Autodesk Inventor part; units mm, degrees
ref_plane "YZ Plane" through (0, 0, 0) normal (1, 0, 0) x (0, 1, 0)
ref_plane "XZ Plane" through (0, 0, 0) normal (0, 1, 0) x (-1, 0, 0)
ref_plane "XY Plane" through (0, 0, 0) normal (0, 0, 1) x (1, 0, 0)
sketch "Sketch1" plane through (0, 0, 0) normal (0, 0, 1) x (1, 0, 0)
  line L0 (107.2618, 7.9599) -> (127.2618, 7.9599)
  line L1 (127.2618, 7.9599) -> (127.2618, 2.9599)
  line L2 (127.2618, 2.9599) -> (107.2618, 2.9599)
  line L3 (107.2618, 2.9599) -> (107.2618, 7.9599)
  circle A0 centre (-95.9382, -3.1699) radius 7.5
  circle A1 centre (-95.9382, -3.1699) radius 10
  line L4 (-95.9382, -13.1699) -> (-67.2988, -13.1699)
  line L5 (-67.2988, -13.1699) -> (17.5278, -13.1699)
  line L6 (107.2618, 2.9599) -> (17.5278, -13.1699)
  line L7 (-95.9382, 6.8301) -> (17.5278, 6.8301)
  line L8 (17.5278, 6.8301) -> (107.2618, 7.9599)
  line L9 (-105.7312, -1.1457) -> (-107.876, -1.1457)
  line L10 (-109.876, -3.1457) -> (-109.876, -3.9908)
  line L11 (-107.876, -5.9908) -> (-105.5321, -5.9908)
  arc A2 (-107.876, -1.1457) -> (-109.876, -3.1457) centre (-107.876, -3.1457) ccw
  arc A3 (-109.876, -3.9908) -> (-107.876, -5.9908) centre (-107.876, -3.9908) ccw
  point P0 (0, 0)
  point P1 (107.2618, 5.4599)
  point P2 (-109.876, -5.9908)
  point P3 (-109.876, -1.1457)
  dimension "d0" = 20
  dimension "d1" = 15
  dimension "d2" = 203.2
  dimension "d3" = 20
  dimension "d4" = 5
  dimension "d43" = 2
extrude "Extrusion1" add sketch "Sketch1" along normal blind 7
sketch "Sketch2" plane through (107.2618, 7.9599, 0) normal (0, 1, 0) x (1, 0, 0)
  line L0 (20, 0) -> (20, -7)
  circle A0 centre (20, -3.5) radius 14
  circle A1 centre (20, -3.5) radius 9.5 construction
  circle A2 centre (20, -3.5) radius 8 construction
  line L1 (20, -3.5) -> (29.8995, 6.3995) construction
  line L2 (20, -3.5) -> (34, -3.5) construction
  line L3 (20, -3.5) -> (10.1005, 6.3995) construction
  line L4 (20, -3.5) -> (10.1005, -13.3995) construction
  line L5 (20, -3.5) -> (29.8995, -13.3995) construction
  point P0 (-107.2618, 0)
  point P1 (13.2825, 3.2175)
  point P2 (26.7175, -10.2175)
  point P3 (25.6569, 2.1569)
  point P4 (14.3431, -9.1569)
  dimension "d7" = 28
  dimension "d8" = 19
  dimension "d9" = 16
  dimension "d10" = 45
extrude "Extrusion2" add sketch "Sketch2" against normal blind 5
hole "Hole1" at (120.5443, 7.9599, -3.2175) at (133.9793, 7.9599, 10.2175) at (132.9187, 7.9599, -2.1569) at (121.605, 7.9599, 9.1569) direction (0, -1, 0) diameter 3 end through all
fillet "Fillet1" radius 6 2 edges at (113.7064, 5.4599, 7) (113.7064, 5.4599, 0)
sketch "Sketch4" plane through (0, 0, 7) normal (0, 0, 1) x (1, 0, 0)
  line L0 (17.5278, 6.8301) -> (-95.9382, 6.8301)
  line L1 (-76.1299, 6.8301) -> (-50.7299, 6.8301) construction
  line L2 (-74.4257, 17.0506) -> (-74.4257, 6.8301)
  line L3 (-76.1299, 6.8301) -> (-74.4257, 6.8301)
  line L4 (-74.4257, 6.8301) -> (-82.4257, 6.8301)
  line L5 (-82.4257, 6.8301) -> (-82.4257, 24.5167)
  line L6 (-74.4257, 17.0506) -> (-82.2594, 24.6356)
  line L7 (-82.2594, 24.6356) -> (-82.4257, 24.5167)
  point P0 (0, 0)
  dimension "d42" = 8
extrude "Extrusion4" add sketch "Sketch4" against normal up to surface (7 mm away)
fillet "Fillet3" radius 8 1 edges at (-74.4257, 6.8301, 3.5)
properties part number "BOOM ARM" material "Aluminum 6061"
Source: CAD feature listing. Evaluate the final solid. Frame: model axes, mm. A direction names the side the tool comes from. Round coordinates to 2 decimals unless told otherwise and drop trailing zeros. Loops run counter-clockwise (first coordinate to the right, second up) from the corner with the lowest first, then second, coordinate; pieces in that order, holes last. Notation, with made-up numbers: M -40,69 L 6,69 A33 ccw 6,106 Z; hole C 82,52 d11. An arc over 180 degrees is marked long. Return JSON: item names as keys, results as strings. Group by question number.
1. Mould query, pull axis X, two halves, no side actions, for faces 1 (the face through (-72.02, 9.11, 3.45)), 2 (the face through (-40, -13.17, 3)), 3 (the face through (-102.33, 4.52, 3.45)), 4 (the face through (-25, 6.83, 3)). Classes: released by +X, released by -X, zero draft, split by the parting line, or undercut.
2. Pin query (flat end, axial travel): pin 1 (7.5 mm diameter, centred on x = -88.5, z = 2, fed in from +Y); pin 2 (8 mm diameter, centred on x = 59.5, z = -7.5, fed in from +Y); pin 3 (1.2 mm diameter, centred on x = -106.5, z = 2.5, fed in from -Y); pin 4 (12 mm diameter, centred on y = 7.5, z = 6, fed in from -X). Return the tip coordinate at first contact, or that it passes through.
3. Section query B-B on z = 3.5. Output: boundary loops of the cut face in (x, y), and give its area (3 significant figures).
4. Section query A-A on x = -92. Output: boundary loops of the cut face in (y, z).
5. Section query D-D on y = 20. Output: boundary loops of the cut face in (x, z).
6. Reachability of faces 5 (the face through (-2, -2, 7)), 6 (the face through (-89, 6.83, 3)), 7 (the face through (-2, -2, 0)) from +Z, -Z, +X, -X, +Y, -Y: full face, straight path, thin tool, end or side. Return the list, or none.
7. Section query C-C on x = -58. Output: boundary loops of the cut face in (y, z), and give its area (3 significant figures).
8. Material intervals for line 1 along Y through (x, z) = (-48, 5.5); line 2 along X through (y, z) = (3.5, 0.5); line 3 along Z through (x, y) = (6.5, 1.5), sorted ascending. Write a range as from..to.
Checks:
{
 "1": {"face 1": "undercut", "face 2": "zero draft", "face 3": "released by -X", "face 4": "undercut"},
 "2": {"pin 1": "stops at y = 6.83", "pin 2": "passes through", "pin 3": "stops at y = -5.99", "pin 4": "stops at x = -104.78"},
 "3": {"outline": "M -109.88,-3.99 A2 ccw -107.88,-5.99 L -105.53,-5.99 A10 ccw -95.94,-13.17 L 17.53,-13.17 L 107.26,2.96 L 141.26,2.96 L 141.26,7.96 L 107.26,7.96 L 17.53,6.83 L -66.43,6.83 A8 cw -74.43,14.83 L -74.43,17.05 L -82.26,24.64 L -82.43,24.52 L -82.43,6.83 L -95.94,6.83 A10 ccw -105.73,-1.15 L -107.88,-1.15 A2 ccw -109.88,-3.15 Z; hole C -95.94,-3.17 d15", "area": "3,690 mm²"},
 "4": {"outline": "M -13.17,0 L -9.55,0 L -9.55,7 L -13.17,7 Z; M 3.21,0 L 6.83,0 L 6.83,7 L 3.21,7 Z"},
 "5": {"outline": "M -82.43,0 L -77.47,0 L -77.47,7 L -82.43,7 Z"},
 "6": {"face 5": "+Z, -X, +Y, -Y", "face 6": "+Z, -Z, -X, +Y", "face 7": "-Z, -X, +Y, -Y"},
 "7": {"outline": "M -13.17,0 L 6.83,0 L 6.83,7 L -13.17,7 Z", "area": "140 mm²"},
 "8": {"line 1": "y = -13.17..6.83", "line 2": "x = -103.39..-99.37, -92.51..140.94", "line 3": "z = 0..7"}
}
